Answer from the drawing. Dimensions are ordinates in mm from the lowest x, y and z of the part. A direction names the side the tool comes from. Round coordinates to 2 decimals unless told otherwise and drop trailing zeros. Order: outer loops, then holes, each group sorted by start corner. A loop starts at its lowest first (then second) coordinate and runs counter-clockwise, first axis right, second up. Notation, with made-up numbers: M -21,84.25 L 12,84.25 A28 ccw 12,103.25 Z; hole C 17,-30 d7. An arc over 180 degrees is marked long. Write item = value, one per line. Start each with the question number.
(1) A cutting plane is placed at A-A, the plane x = 224. Determine the outline of the cut face in (y, z), and give its area (3 significant figures).
(2) Which of the six approach directions +Z, -Z, +X, -X, +Y, -Y give full straight-line access (tool end or side, diameter ignored) to the marked faces 4, 5 and 6?
(3) For a pull along Y with two mould halves and no side action, classify the marked faces 1, 2 and 3 as released by +Y, released by -Y, zero draft, split by the parting line, or undercut.
(4) Straight lines are drawn through the part: probe 1 along Y at (x, z) = (183, 274); probe 2 along Z at (x, y) = (60.5, 206). For each, find the intervals that lie inside material, in ascending order. Write a range as from..to.
(5) A cutting plane is placed at C-C, the plane z = 254. Determine the outline of the cut face in (x, y), and give its area (3 significant figures).
(6) A cutting plane is placed at D-D, the plane x = 338. Determine the outline of the cut face in (y, z), and give its area (3 significant figures).
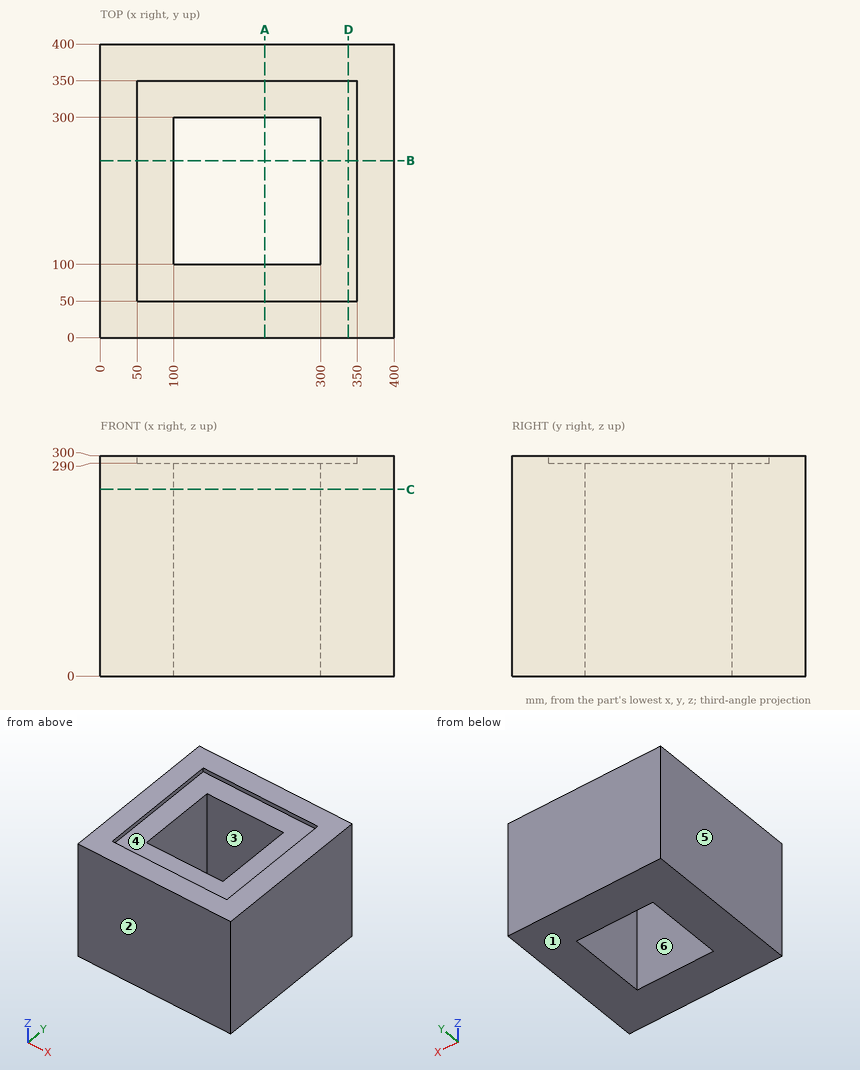
Reported:
q1.outline = M 0,0 L 100,0 L 100,290 L 50,290 L 50,300 L 0,300 Z; M 300,0 L 400,0 L 400,300 L 350,300 L 350,290 L 300,290 Z
q1.area = 59,000 mm²
q2.face_4 = +Z
q2.face_5 = +Z, -Z, -X, +Y, -Y
q2.face_6 = +Z, -Z
q3.face_1 = zero draft
q3.face_2 = released by -Y
q3.face_3 = undercut
q4.probe_1 = 0..100, 300..400
q4.probe_2 = 0..290
q5.outline = M 0,0 L 400,0 L 400,400 L 0,400 Z; hole M 100,100 L 300,100 L 300,300 L 100,300 Z
q5.area = 120,000 mm²
q6.outline = M 0,0 L 400,0 L 400,300 L 350,300 L 350,290 L 50,290 L 50,300 L 0,300 Z
q6.area = 117,000 mm²
